```python
from build123d import *

# Parameters (mm, degrees)
CYLINDER_R                    = 4
CYLINDER_DEPTH                = 2
CYLINDER004_R                 = 0.7
CYLINDER004_DEPTH             = 15
CYLINDER005_R                 = 0.7
CYLINDER005_DEPTH             = 15
CYLINDER006_R                 = 0.7
CYLINDER006_DEPTH             = 15
CYLINDER007_R                 = 0.7
CYLINDER007_DEPTH             = 15
CYLINDER008_R                 = 0.7
CYLINDER008_DEPTH             = 15
CYLINDER009_R                 = 0.7
CYLINDER009_DEPTH             = 15
CYLINDER010_R                 = 0.7
CYLINDER010_DEPTH             = 15
CYLINDER003_R                 = 0.7
CYLINDER003_DEPTH             = 15
CUBE_W                        = 10
CUBE_H                        = 5
CUBE_DEPTH                    = 12
CYLINDER011_R                 = 3.2
CYLINDER011_DEPTH             = 12
CUBE001_W                     = 10
CUBE001_H                     = 5
CUBE001_DEPTH                 = 8
CYLINDER012_R                 = 3.2
CYLINDER012_DEPTH             = 2
CYLINDER002_R                 = 0.5
CYLINDER002_DEPTH             = 6.5
CYLINDER001_R                 = 4.5
CYLINDER001_DEPTH             = 2
REFINEROTATEEXTRUDE_R         = 2
ROTATEEXTRUDE_PLACEMENT_ANGLE = 90
CYLINDER_R_2                  = 6.5
CYLINDER_DEPTH_2              = 15


with BuildPart() as cylinder:
    # Cylinder → Cylinder (new body)
    with BuildSketch(Plane.XY):
        Circle(CYLINDER_R)
    extrude(amount=CYLINDER_DEPTH)


with BuildPart() as cylinder004:
    # cylinder004 → cylinder004 (new body)
    with BuildSketch(Plane(origin=(6.28238, 2.60225, 3), x_dir=(1, 0, 0), z_dir=(0, 0, 1))):
        Circle(CYLINDER004_R)
    extrude(amount=CYLINDER004_DEPTH)


with BuildPart() as cylinder005:
    # cylinder005 → cylinder005 (new body)
    with BuildSketch(Plane(origin=(6.28238, -2.60225, 3), x_dir=(1, 0, 0), z_dir=(0, 0, 1))):
        Circle(CYLINDER005_R)
    extrude(amount=CYLINDER005_DEPTH)


with BuildPart() as cylinder006:
    # cylinder006 → cylinder006 (new body)
    with BuildSketch(Plane(origin=(2.60225, -6.28238, 3), x_dir=(1, 0, 0), z_dir=(0, 0, 1))):
        Circle(CYLINDER006_R)
    extrude(amount=CYLINDER006_DEPTH)


with BuildPart() as cylinder007:
    # cylinder007 → cylinder007 (new body)
    with BuildSketch(Plane(origin=(-2.60225, -6.28238, 3), x_dir=(1, 0, 0), z_dir=(0, 0, 1))):
        Circle(CYLINDER007_R)
    extrude(amount=CYLINDER007_DEPTH)


with BuildPart() as cylinder008:
    # cylinder008 → cylinder008 (new body)
    with BuildSketch(Plane(origin=(-6.28238, -2.60225, 3), x_dir=(1, 0, 0), z_dir=(0, 0, 1))):
        Circle(CYLINDER008_R)
    extrude(amount=CYLINDER008_DEPTH)


with BuildPart() as cylinder009:
    # cylinder009 → cylinder009 (new body)
    with BuildSketch(Plane(origin=(-6.28238, 2.60225, 3), x_dir=(1, 0, 0), z_dir=(0, 0, 1))):
        Circle(CYLINDER009_R)
    extrude(amount=CYLINDER009_DEPTH)


with BuildPart() as cylinder010:
    # cylinder010 → cylinder010 (new body)
    with BuildSketch(Plane(origin=(-2.60225, 6.28238, 3), x_dir=(1, 0, 0), z_dir=(0, 0, 1))):
        Circle(CYLINDER010_R)
    extrude(amount=CYLINDER010_DEPTH)


with BuildPart() as group:
    # cylinder003 → cylinder003 (new body)
    with BuildSketch(Plane(origin=(2.60225, 6.28238, 3), x_dir=(1, 0, 0), z_dir=(0, 0, 1))):
        Circle(CYLINDER003_R)
    extrude(amount=CYLINDER003_DEPTH)

    # Group: union cylinder004, cylinder005, cylinder006, cylinder007, cylinder008, cylinder009, cylinder010
    add(cylinder004.part)
    add(cylinder005.part)
    add(cylinder006.part)
    add(cylinder007.part)
    add(cylinder008.part)
    add(cylinder009.part)
    add(cylinder010.part)


with BuildPart() as cube:
    # cube → cube (new body)
    with BuildSketch(Plane(origin=(-5, -6.6, 2), x_dir=(1, 0, 0), z_dir=(0, 0, 1))):
        with Locations((5, 2.5)):
            Rectangle(CUBE_W, CUBE_H)
    extrude(amount=CUBE_DEPTH)


with BuildPart() as difference:
    # cylinder011 → cylinder011 (new body)
    with BuildSketch(Plane.XY.offset(2)):
        Circle(CYLINDER011_R)
    extrude(amount=CYLINDER011_DEPTH)

    # difference: cut cube
    add(cube.part, mode=Mode.SUBTRACT)


with BuildPart() as cube001:
    # cube001 → cube001 (new body)
    with BuildSketch(Plane(origin=(-5, -6.6, 0), x_dir=(1, 0, 0), z_dir=(0, 0, 1))):
        with Locations((5, 2.5)):
            Rectangle(CUBE001_W, CUBE001_H)
    extrude(amount=CUBE001_DEPTH)


with BuildPart() as difference001:
    # cylinder012 → cylinder012 (new body)
    with BuildSketch(Plane.XY):
        Circle(CYLINDER012_R)
    extrude(amount=CYLINDER012_DEPTH)

    # difference001: cut cube001
    add(cube001.part, mode=Mode.SUBTRACT)


with BuildPart() as union001:
    # cylinder002 → cylinder002 (new body)
    with BuildSketch(Plane(origin=(0, 0, 17), x_dir=(1, 0, 0), z_dir=(0, 1, 0))):
        Circle(CYLINDER002_R)
    extrude(amount=CYLINDER002_DEPTH)

    # union001: union Group, difference, difference001
    add(group.part)
    add(difference.part)
    add(difference001.part)


with BuildPart() as cylinder001:
    # cylinder001 → cylinder001 (new body)
    with BuildSketch(Plane.XY.offset(15)):
        Circle(CYLINDER001_R)
    extrude(amount=CYLINDER001_DEPTH)


with BuildPart() as rotateextrude:
    # RefineRotateExtrude → RotateExtrude (revolve)
    with BuildSketch(Plane(origin=(4.5, 0, 0), x_dir=(0, 1, 0), z_dir=(0, 0, 1))):
        Circle(REFINEROTATEEXTRUDE_R)
    revolve(axis=Axis((0, 0, 0), (0, 1, 0)))


with BuildPart() as rotateextrude_1:
    # RotateExtrude placement: moved
    add(rotateextrude.part.moved(Location((0, 0, 15))).rotate(Axis((0, 0, 15), (1, 0, 0)), ROTATEEXTRUDE_PLACEMENT_ANGLE))


with BuildPart() as cut:
    # cylinder → cylinder (new body)
    with BuildSketch(Plane.XY):
        Circle(CYLINDER_R_2)
    extrude(amount=CYLINDER_DEPTH_2)

    # union: union cylinder001, RotateExtrude
    add(cylinder001.part)
    add(rotateextrude_1.part)

    # difference002: cut union001
    add(union001.part, mode=Mode.SUBTRACT)

    # Cut: cut Cylinder
    add(cylinder.part, mode=Mode.SUBTRACT)


solid = cut.part
```
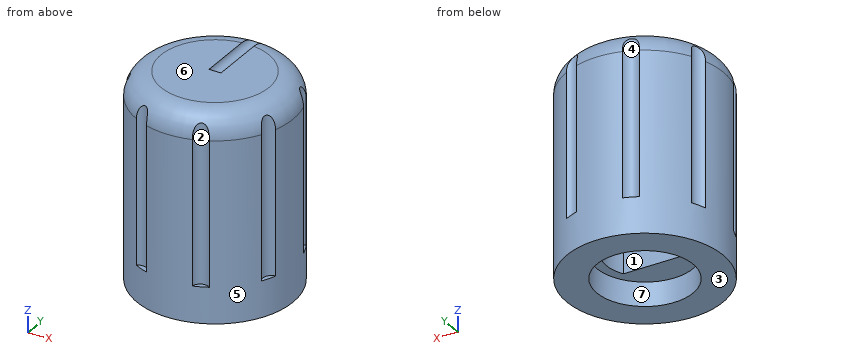
The listing builds one solid part. Answer for the finished solid, in the listing's coordinates (mm). Face numbers are marked on the shaded views. A direction names the side the tool comes from. Give positions to 0.01 mm unless a question says otherwise; leave off trailing zeros. Order: outer loops, then holes, each group sorted by start corner. A loop starts at its lowest first (then second) coordinate and runs counter-clockwise, first axis right, second up.
Item 1: The part is cut by section B-B, the plane x = 0. Give the vertices of the cut face in (y, z), and give its area (3 significant figures).
From the geometry:
outline: (-6.5, 0) - (-4, 0) - (-4, 2) - (-1.6, 2) - (-1.6, 14) - (3.2, 14) - (3.2, 2) - (4, 2) - (4, 0) - (6.5, 0) - (6.5, 15) arc R2 ccw to (5.82, 16.5) - (0, 16.5) - (0, 17) - (-4.5, 17) arc R2 ccw to (-6.5, 15) - close
area: 143 mm2
Item 2: Given pin 1 Ø0.5 at (x, y) = (2.5, -6) entering from +Z; pin 2 Ø6.5 at (x, y) = (0.5, -1.5) entering from -Z; pin 3 Ø2.5 at (x, y) = (-1, 1) entering from -Z; pin 4 Ø6 at (x, y) = (0, 0) entering from -Z, each flat-ended and moving along its own axis, determine where each tip first touches the part or whether it passes through.
From the geometry:
pin 1: stops at z = 3
pin 2: stops at z = 0
pin 3: stops at z = 14
pin 4: stops at z = 2
Item 3: Find the intervals of material crossed by probe 1 along Y at (x, z) = (0, 1.3); probe 2 along X at (y, z) = (2.75, 0.5); probe 3 along Z at (x, y) = (2.5, -1.75), in increasing order.
From the geometry:
probe 1: y = -6.5 to -4, 4 to 6.5
probe 2: x = -5.89 to -2.9, 2.9 to 5.89
probe 3: z = 2 to 17
Item 4: The part is cut by section A-A, the plane z = 13.75. Give the vertices of the cut face in (x, y), and give its area (3 significant figures).
From the geometry:
outline: (-6.21, -1.91) arc R0.7 cw to (-5.74, -3.05) arc R6.5 ccw to (-3.05, -5.74) arc R0.7 cw to (-1.91, -6.21) arc R6.5 ccw to (1.91, -6.21) arc R0.7 cw to (3.05, -5.74) arc R6.5 ccw to (5.74, -3.05) arc R0.7 cw to (6.21, -1.91) arc R6.5 ccw to (6.21, 1.91) arc R0.7 cw to (5.74, 3.05) arc R6.5 ccw to (3.05, 5.74) arc R0.7 cw to (1.91, 6.21) arc R6.5 ccw to (-1.91, 6.21) arc R0.7 cw to (-3.05, 5.74) arc R6.5 ccw to (-5.74, 3.05) arc R0.7 cw to (-6.21, 1.91) arc R6.5 ccw to start; hole (-2.77, -1.6) - (2.77, -1.6) arc R3.2 ccw (long way) to start
area: 104 mm2
Item 5: For a pull along Y with two mould halves and no side action, classify the marked faces 4, 5, 6 and 7 as pulls with the +Y half, pulls with the -Y half, needs draft (parallel to the pull), parting line crosses it, or undercut.
From the geometry:
face 4: pulls with the +Y half
face 5: parting line crosses it
face 6: needs draft
face 7: undercut
Item 6: Which of the six approach directions +Z, -Z, +X, -X, +Y, -Y give full straight-line access (tool end or side, diameter ignored) to the marked faces 1, 2 and 3?
From the geometry:
face 1: -Z
face 2: +Z, -Y
face 3: -Z, +X, -X, +Y, -Y
